from build123d import *

# Parameters (mm, degrees)
EXTRUDE_4_DEPTH = 15


with BuildPart() as part:
    # Эскиз8 → Бобышка-Вытянуть4 (new body)
    with BuildSketch(Plane.XY):
        Polygon((0, 0), (0, 11), (-0.7, 14.71), (-3.7, 14.71), (-4.4, 11), (-7.4, 11), (-8.1, 14.71), (-11.1, 14.71), (-11.8, 11), (-14.8, 11), (-15.5, 14.71), (-18.5, 14.71), (-19.2, 11), (-22.2, 11), (-22.9, 14.71), (-25.9, 14.71), (-26.6, 11), (-29.6, 11), (-30.3, 14.71), (-33.3, 14.71), (-34, 11), (-37, 11), (-37.7, 14.71), (-40.7, 14.71), (-41.4, 11), (-44.4, 11), (-45.1, 14.71), (-48.1, 14.71), (-48.8, 11), (-51.8, 11), (-52.5, 14.71), (-55.5, 14.71), (-56.2, 11), (-59.2, 11), (-59.9, 14.71), (-62.9, 14.71), (-63.6, 11), (-66.6, 11), (-67.3, 14.71), (-70.3, 14.71), (-71, 11), (-74, 11), (-74.7, 14.71), (-77.7, 14.71), (-78.4, 11), (-81.4, 11), (-82.1, 14.71), (-85.1, 14.71), (-85.8, 11), (-88.8, 11), (-89.5, 14.71), (-92.5, 14.71), (-93.2, 11), (-96.2, 11), (-96.240718782, 0), align=None)
    extrude(amount=EXTRUDE_4_DEPTH)


solid = part.part
Could you check a few things on this model? Use its own coordinates, in mm. A direction names the side the tool comes from. Coordinates: 2 decimals unless noted, no trailing zeros. One line per question, with ' | ' between items.
Q1. On a 3-axis mill with a long thin cutter (end or side, diameter ignored), from which of +Z, -Z, +X, -X, +Y, -Y can I reach the whole of each face in a straight line? I mean faces 5 (the face through (-6, 11, 7)), 6 (the face through (-32, 14.71, 7)). Say none if no direction works.
Return value:
face 5: +Z, -Z, +Y | face 6: +Z, -Z, +X, -X, +Y
Q2. Imagine slicing it at A-A on y = 13.5. State how many separate pieces and enclosed holes the cut face has, and give its area (3 significant figures).
Return value:
separate pieces: 13 | enclosed holes: 0 | area: 674 mm²
Q3. If I drill on L1, parallel to Y at x = -59, z = 3.5; L2, parallel to X at y = 2.75, z = 9.25, over which ranges is the centre line in solid material (lowest first)?
Return value:
L1: 0 to 11 | L2: -96.23 to 0
Q4. I'm going to push flat-ended pins straight in: P1, Ø0.9, axis at x = -65.5, z = 6.5, coming from the +Y side; P2, Ø2, axis at y = 4, z = 13, coming from the -X side. Where does each tip first touch, or does it pass through?
Return value:
P1: y = 11 | P2: x = -96.23
Q5. Thinking about a two-plate mould opening in X: for faces 1 (the face through (-13, 11, 7)), 2 (the face through (-39, 14.71, 7)), 3 (the face through (-92.845, 12.881, 7.395)), 4 (the face through (-89.145, 12.829, 7.395)), which applies, pulls with the +X half, pulls with the -X half, needs draft (parallel to the pull), parting line crosses it, or undercut?
Return value:
face 1: undercut | face 2: needs draft | face 3: pulls with the -X half | face 4: undercut
